Design review of the part built by this model. Coordinates are the model's own, in mm. Face numbers are marked on the shaded views. Coordinates: 2 decimals unless noted, no trailing zeros. Write each loop counter-clockwise with the first axis right and the second up, starting at its lowest first coordinate (ties: lowest second). Pieces come first, ordered by that corner, then holes. Notation, with made-up numbers: M 63,67 L 109,67 A25 ccw 109,102 Z; hole C 29,-39 d2. An arc over 180 degrees is marked long. Write item = value, one per line.
```python
from build123d import *

# Parameters (mm, degrees)
SHELL1_OUTLINE_R     = 25
SHELL1_DEPTH         = 122.5
SHELL1_2_OUTLINE_R   = 32.5
SHELL1_2_OUTLINE_R_2 = 25
SHELL1_2_DEPTH       = 7.5
SHELL1_START         = 117
SHELL1_3_OUTLINE_R   = 27.5
SHELL1_3_OUTLINE_R_2 = 25
SHELL1_3_DEPTH       = 5.5
FILLET1_R            = 10
FILLET2_R            = 10


# Read off the part's stored shape, not the designer's step: Shell1
with BuildPart() as part:
    # Sketch1 → Revolve1 (revolve)
    with BuildSketch(Plane(origin=(0, 0, 0), x_dir=(1, 0, 0), z_dir=(0, 1, 0)), mode=Mode.PRIVATE) as revolve1_sk:
        Polygon((0, 0), (0, -122.5), (30, -122.5), (30, -119.5), (32.5, -119.5), (32.5, -114.5), (27.5, -114.5), (27.5, -10), (37.5, -10), (37.5, -5), (35, -5), (35, 0), align=None)
    revolve(revolve1_sk.sketch.rotate(Axis((0, 0, 0), (0, 0, 1)), 180), axis=Axis((0, 0, 0), (0, 0, 1)))

    # Shell1 outline → Shell1 (cut)
    with BuildSketch(Plane.XY):
        Circle(SHELL1_OUTLINE_R)
    extrude(amount=SHELL1_DEPTH, mode=Mode.SUBTRACT)

    # Shell1 2 outline → Shell1 2 (cut)
    with BuildSketch(Plane.XY):
        Circle(SHELL1_2_OUTLINE_R)
        Circle(SHELL1_2_OUTLINE_R_2, mode=Mode.SUBTRACT)
    extrude(amount=SHELL1_2_DEPTH, mode=Mode.SUBTRACT)

    # Shell1 3 outline → Shell1 3 (cut)
    with BuildSketch(Plane.XY.offset(SHELL1_START)):
        Circle(SHELL1_3_OUTLINE_R)
        Circle(SHELL1_3_OUTLINE_R_2, mode=Mode.SUBTRACT)
    extrude(amount=SHELL1_3_DEPTH, mode=Mode.SUBTRACT)

    # Fillet1
    # the kernel refuses this fillet: 10 mm, written as the material it adds along each edge
    with BuildSketch(Plane(origin=(0, 0, 10), x_dir=(-1, 0, 0), z_dir=(0, 1, 0))) as fillet1_piece_1:
        with BuildLine():
            CenterArc((27.5 + FILLET1_R, FILLET1_R), FILLET1_R, 180, 90)
            Line((27.5 + FILLET1_R, 0), (27.5 + FILLET1_R, -FILLET1_R * 0.02))
            Line((27.5 + FILLET1_R, -FILLET1_R * 0.02), (27.5 - FILLET1_R * 0.02, -FILLET1_R * 0.02))
            Line((27.5 - FILLET1_R * 0.02, -FILLET1_R * 0.02), (27.5 - FILLET1_R * 0.02, FILLET1_R))
            Line((27.5 - FILLET1_R * 0.02, FILLET1_R), (27.5, FILLET1_R))
        make_face()
    revolve(axis=Axis((0, 0, 10), (0, 0, 1)))
    with BuildSketch(Plane(origin=(0, 0, 114.5), x_dir=(-1, 0, 0), z_dir=(0, 1, 0))) as fillet1_piece_2:
        with BuildLine():
            CenterArc((37.5, -8.660254038), FILLET1_R, 120, 60)
            Line((27.5, -8.660254038), (27.3, -8.660254038))
            Line((27.3, -8.660254038), (27.3, 0))
            Line((27.3, 0), (27.5, 0.2))
            ThreePointArc((27.5, 0.2), (30, 0.2), (32.4, 0.173205081))
            Line((32.4, 0.173205081), (32.5, 0))
        make_face()
    revolve(axis=Axis((0, 0, 114.5), (0, 0, 1)))

    # Fillet2
    # the kernel refuses this fillet: 10 mm, written as the material it takes off along each edge
    with BuildSketch(Plane(origin=(0, 0, 10), x_dir=(-1, 0, 0), z_dir=(0, 1, 0))) as fillet2_piece_1:
        with BuildLine():
            CenterArc((27.817541634, -7.5), FILLET2_R, 14.477512186, 46.567463442)
            Line((37.5, -5), (37.693649167, -4.95))
            ThreePointArc((37.693649167, -4.95), (37.7, -2.5), (37.7, 0))
            Line((37.7, 0), (37.5, 0.2))
            ThreePointArc((37.5, 0.2), (35.05, 0.511190802), (32.755595401, 1.425))
            Line((32.755595401, 1.425), (32.658770817, 1.25))
        make_face()
    revolve(axis=Axis((0, 0, 10), (0, 0, 1)), mode=Mode.SUBTRACT)
    with BuildSketch(Plane(origin=(0, 0, 114.5), x_dir=(-1, 0, 0), z_dir=(0, 1, 0))) as fillet2_piece_2:
        with BuildLine():
            CenterArc((22.5, 4.568502517), FILLET2_R, 318.590377891, 41.409622109)
            Line((32.5, 4.568502517), (32.7, 4.568502517))
            Line((32.7, 4.568502517), (32.7, 0))
            Line((32.7, 0), (32.6, -0.173205081))
            ThreePointArc((32.6, -0.173205081), (31.293504258, -1.076098804), (30.15, -2.178163326))
            Line((30.15, -2.178163326), (30, -2.04587576))
        make_face()
    revolve(axis=Axis((0, 0, 114.5), (0, 0, 1)), mode=Mode.SUBTRACT)


solid = part.part
```
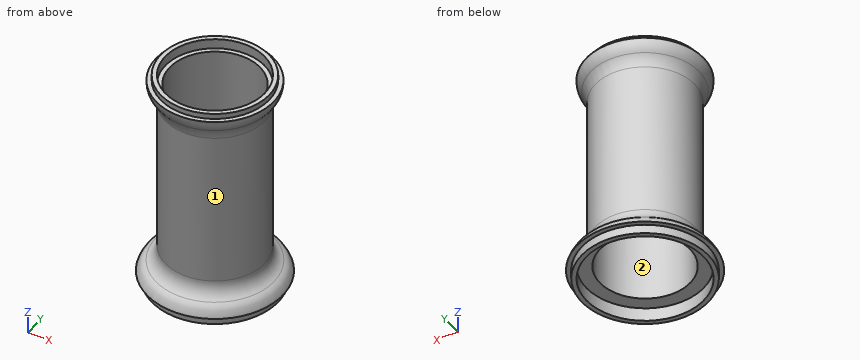
Q1. Wall thickness on line 1 (Y direction, x = 0, z = 118.85); line 2 (X direction, y = -6.5, z = 99.5); line 3 (Z direction, x = 7.5, y = -25): over which ranges is each line inside the solid? List them lowest first.
Check result:
line_1 = -32.5 to -27.5, 27.5 to 32.5
line_2 = -26.72 to -24.14, 24.14 to 26.72
line_3 = 7.5 to 117
Q2. The part is to be moulded in two halves that separate along X. For the marked faces 1 and 2, say which applies: +X half, -X half, draft (parallel to the pull), parting line (faces both ways), or undercut.
Check result:
face_1 = parting line
face_2 = undercut
Q3. For P1, Ø8, axis at x = 1.5, z = 47, coming from the -Y side; P2, Ø5, axis at x = 20, z = 58.5, coming from the +Y side; P3, Ø8, axis at x = -8, z = 24, coming from the -Y side, all flat-tipped, find the tip position at first contact; note any pin that passes through.
Check result:
P1 = -27.5
P2 = 21.21
P3 = -27.21
Q4. Consider section D-D, the plane z = 15.5. State the section outline as (x, y) points, and give its area (3 significant figures).
Check result:
outline = C 0,0 d57.14; hole C 0,0 d50
area = 601 mm²
Q5. Consider section C-C, the plane z = 83. State the section outline as (x, y) points, and give its area (3 significant figures).
Check result:
outline = C 0,0 d55; hole C 0,0 d50
area = 412 mm²
